from build123d import *

# Parameters (mm, degrees)
F0_W     = 113.953635
F0_H     = 72.534319
F0_R     = 5.859318
F1_DEPTH = 25.4
F2_DEPTH = 30.48


with BuildPart() as f1:
    # F0 (on Front) → F1 (new body)
    with BuildSketch(Plane.XZ):
        with Locations((7.273636, -2.727615)):
            Rectangle(F0_W, F0_H)
        with Locations((-33.539545, 17.78)):
            Circle(F0_R, mode=Mode.SUBTRACT)
        Polygon((-4.753076, 29.036522), (-1.770401, 23.004169), (-5.503234, 17.40492), (-12.218743, 17.838024), (-15.201418, 23.870377), (-11.468585, 29.469626), align=None, mode=Mode.SUBTRACT)
    extrude(amount=F1_DEPTH)

    # F0 (on Front) → F2 (join)
    with BuildSketch(Plane.XZ):
        with Locations((-33.539545, 17.78)):
            Circle(F0_R)
    extrude(amount=F2_DEPTH)


solid = f1.part
Design review of the part built by this model. Coordinates are the model's own, in mm. A direction names the side the tool comes from. Round coordinates to 2 decimals unless told otherwise and drop trailing zeros. Write each loop counter-clockwise with the first axis right and the second up, starting at its lowest first coordinate (ties: lowest second). Pieces come first, ordered by that corner, then holes. Notation, with made-up numbers: (38.25, 48.5) - (42.25, 48.5) arc R9 ccw to (42.25, 58.5) - close; hole circle Ø8 at (-3, 80). An arc over 180 degrees is marked (long way). Use a Markdown table: item, result. Add a question column.
1. We need section B-B (x = 30.5). State the section outline as (y, z) points.
2. Clearance check with a flat-ended pin moving along its axis: pin 1 (4 mm diameter, centred on x = -35, z = -2, fed in from -Y). State where the tip first meets the part, or that it passes through.
3. Mouldability with a two-part tool opening along X and no side actions: class faces 4 (the face through (64.25, -13, -3)), 5 (the face through (-49.703, -13, -3)), 6 (the face through (-3.611, -12.522, 20.244)) as +X half, -X half, draft (parallel to the pull), parting line (faces both ways), or undercut.
4. Wall thickness on probe 1 along X at (y, z) = (-23, 27.5); probe 2 along Y at (x, z) = (39.5, 1.5); probe 3 along X at (y, z) = (-10, 28.5) (3 decimals): over which ranges is each line inside the solid? List them lowest first.
5. For faces 1 (the face through (-8.158, -12.522, 29.256)), 2 (the face through (6, -13, 33.54)), 3 (the face through (-27.95, -27.9, 19.54)), list the 3-axis set-ups (+Z, -Z, +X, -X, +Y, -Y) from which the entire face can be reached by the end or side of a thin tool; tool diameter is ignored.
6. We need section A-A (z = 5). State the section outline as (x, y) points, then the cut area to 3 significant figures.
Output:
| question | item | result |
|---|---|---|
| 1 | outline | (-25.4, -38.99) - (0, -38.99) - (0, 33.54) - (-25.4, 33.54) - close |
| 2 | pin 1 | stops at y = -25.4 |
| 3 | face 4 | +X half |
| 3 | face 5 | -X half |
| 3 | face 6 | undercut |
| 4 | probe 1 | x = -49.7 to -12.78, -3.99 to 64.25 |
| 4 | probe 2 | y = -25.4 to 0 |
| 4 | probe 3 | x = -49.703 to -12.115, -4.488 to 64.25 |
| 5 | face 1 | +Y, -Y |
| 5 | face 2 | +Z, +X, -X, +Y, -Y |
| 5 | face 3 | -Y |
| 6 | outline | (-49.7, -25.4) - (64.25, -25.4) - (64.25, 0) - (-49.7, 0) - close |
| 6 | area | 2,890 mm2 |
